```python
from build123d import *

# Parameters (mm, degrees)
Y_KSEKLIK_EKSTR_ZYON1_DEPTH = 4
IZIM2_W                     = 4
IZIM2_H                     = 27
Y_KSEKLIK_EKSTR_ZYON2_DEPTH = 44.221383782
Y_KSEKLIK_EKSTR_ZYON3_REACH = 97.396
IZIM3_W                     = 3.790620303
IZIM3_H                     = 20.022795238
IZIM4_W                     = 3.790620303
IZIM4_H                     = 47
Y_KSEKLIK_EKSTR_ZYON4_DEPTH = 16
IZIM5_W                     = 3.790620303
IZIM5_H                     = 47
Y_KSEKLIK_EKSTR_ZYON5_DEPTH = 18.977204763
IZIM6_W                     = 40
IZIM6_H                     = 40
KES_EKSTR_ZYON1_DEPTH       = 111.308229444
F_23_0_23_AP_DELIK1_D       = 23
F_4_0_4_AP_DELIK1_D         = 4
F_4_0_4_AP_DELIK1_DEPTH     = 56.792653887


with BuildPart() as part:
    # Çizim1 → Yükseklik-Ekstrüzyon1 (new body)
    with BuildSketch(Plane.XY.offset(4)):
        with BuildLine():
            Line((-27.146814404, 25.956036228), (-27.146814404, -25.956036228))
            ThreePointArc((-27.146814404, -25.956036228), (-26.258437345, -27.618652972), (-24.382519966, -27.804239142))
            Line((-24.382519966, -27.804239142), (38.383894912, -1.848202914))
            ThreePointArc((38.383894912, -1.848202914), (39.619600474, 0), (38.383894912, 1.848202914))
            Line((38.383894912, 1.848202914), (-24.382519966, 27.804239142))
            ThreePointArc((-24.382519966, 27.804239142), (-26.258437345, 27.618652972), (-27.146814404, 25.956036228))
        make_face()
    extrude(amount=-Y_KSEKLIK_EKSTR_ZYON1_DEPTH)

    # Çizim2 → Yükseklik-Ekstrüzyon2 (add)
    with BuildSketch(Plane.ZY.offset(27.146814404)):
        with Locations((2, 0.476036228)):
            Rectangle(IZIM2_W, IZIM2_H)
    extrude(amount=Y_KSEKLIK_EKSTR_ZYON2_DEPTH)

    # Çizim3 → Yükseklik-Ekstrüzyon3 (add, up to next)
    with BuildSketch(Plane.XY.offset(56.792653887), mode=Mode.PRIVATE) as y_kseklik_ekstr_zyon3_sk1:
        with Locations((16.748495748, 0)):
            Rectangle(IZIM3_W, IZIM3_H)
    y_kseklik_ekstr_zyon3_tool1 = extrude(y_kseklik_ekstr_zyon3_sk1.sketch, amount=-Y_KSEKLIK_EKSTR_ZYON3_REACH, mode=Mode.PRIVATE) - part.part
    add(y_kseklik_ekstr_zyon3_tool1.solids().sort_by_distance((16.748496, 0, 56.792654))[0])

    # Çizim4 → Yükseklik-Ekstrüzyon4 (add)
    with BuildSketch(Plane(origin=(0, 10.011397619, 0), x_dir=(-1, 0, 0), z_dir=(0, 1, 0))):
        with Locations((-16.748495748, 33.292653887)):
            Rectangle(IZIM4_W, IZIM4_H)
    extrude(amount=Y_KSEKLIK_EKSTR_ZYON4_DEPTH)

    # Çizim5 → Yükseklik-Ekstrüzyon5 (add)
    with BuildSketch(Plane.XZ.offset(10.011397619)):
        with Locations((16.748495748, 33.292653887)):
            Rectangle(IZIM5_W, IZIM5_H)
    extrude(amount=Y_KSEKLIK_EKSTR_ZYON5_DEPTH)

    # Çizim6 → Kes-Ekstrüzyon1 (cut, through all)
    with BuildSketch(Plane(origin=(18.643805899, 0, 0), x_dir=(0, 0, -1), z_dir=(1, 0, 0))):
        with Locations((-33.968638069, -1.488602381)):
            Rectangle(IZIM6_W, IZIM6_H)
    extrude(amount=-KES_EKSTR_ZYON1_DEPTH, mode=Mode.SUBTRACT)

    # Ø23.0 (23) Çap Delik1 (through all)
    with Locations(Plane.XY.offset(4)):
        with Locations((-58.625359309, 0.476036228)):
            Hole(F_23_0_23_AP_DELIK1_D / 2)

    # Ø4.0 (4) Çap Delik1
    with Locations(Plane(origin=(0, 0, 0), x_dir=(-1, 0, 0), z_dir=(0, 0, -1))):
        with Locations((23.146814404, -22.964704035), (23.146814404, 22.964704035), (-32.386015353, 0)):
            Hole(F_4_0_4_AP_DELIK1_D / 2, depth=F_4_0_4_AP_DELIK1_DEPTH)


solid = part.part
```
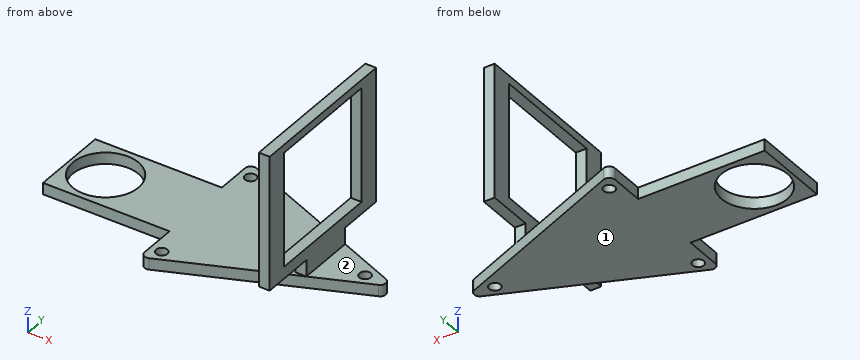
Verification items for the finished model (mm, model axes). Face numbers are marked on the shaded views. A direction names the side the tool comes from. Round coordinates to 2 decimals unless told otherwise and drop trailing zeros. Write each loop counter-clockwise with the first axis right and the second up, starting at its lowest first coordinate (ties: lowest second). Pieces come first, ordered by that corner, then holes. Notation, with made-up numbers: (75.25, 80) -> (127.25, 80) arc R8 cw to (127.25, 85) -> close; hole circle Ø6 at (68.5, -6). An arc over 180 degrees is marked (long way). Write each question's results on one line, items separated by ' | '. Start each with the question number.
1. Material ranges on probe 1 along Z at (x, y) = (16.5, 15); probe 2 along X at (y, z) = (22.5, 11.5); probe 3 along Z at (x, y) = (25, -6.5), recorded low to high. Write a range as from..to.
2. Depth check by flat-ended pin: P1, Ø4, axis at x = 16.5, y = -17, coming from the -Z side; P2, Ø3, axis at x = 17.5, z = 7, coming from the +Y side; P3, Ø2, axis at x = -51.5, z = 1, coming from the +Y side. Enter the tip coordinate at first touch or a pass-through.
3. Cross-section at A-A (z = 42.5). Enter the section's corners in (x, y), then the cut area to 3 significant figures.
4. Cross-section at D-D (z = 11). Enter the section's corners in (x, y).
5. Cross-section at B-B (y = -19). Enter the section's corners in (x, z).
6. Cross-section at C-C (x = -32). Enter the section's corners in (y, z), then the cut area to 3 significant figures.
7. Set-up check for the marked faces 1 and 2: record each of +Z, -Z, +X, -X, +Y, -Y from which the full face is reachable in a straight line by a thin tool's end or side.
Solutions:
1) probe 1: z = 9.79..13.97, 53.97..56.79 | probe 2: x = 14.85..18.64 | probe 3: z = 0..4
2) P1: stops at z = 9.79 | P2: stops at y = 10.01 | P3: stops at y = 13.98
3) outline: (14.85, -28.99) -> (18.64, -28.99) -> (18.64, -21.49) -> (14.85, -21.49) -> close; (14.85, 18.51) -> (18.64, 18.51) -> (18.64, 26.01) -> (14.85, 26.01) -> close | area: 56.9 mm2
4) outline: (14.85, -28.99) -> (18.64, -28.99) -> (18.64, 26.01) -> (14.85, 26.01) -> close
5) outline: (-27.15, 0) -> (-3.09, 0) -> (-3.09, 4) -> (-27.15, 4) -> close; (14.85, 9.79) -> (18.64, 9.79) -> (18.64, 13.97) -> (14.85, 13.97) -> close; (14.85, 53.97) -> (18.64, 53.97) -> (18.64, 56.79) -> (14.85, 56.79) -> close
6) outline: (-13.02, 0) -> (13.98, 0) -> (13.98, 4) -> (-13.02, 4) -> close | area: 108 mm2
7) face 1: -Z, +X, -X, +Y, -Y | face 2: +Z, +X, +Y, -Y
